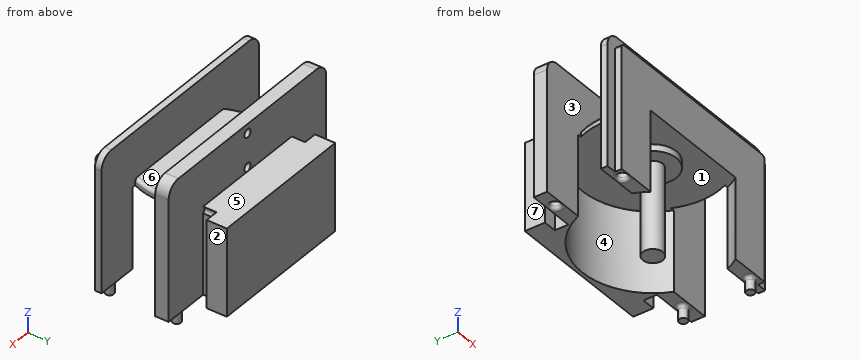
```python
from build123d import *

# Parameters (mm, degrees)
BOSS_EXTRUDE1_DEPTH     = 1
SKETCH2_R               = 1.475
BOSS_EXTRUDE2_DEPTH     = 14
SKETCH3_R               = 3.5
BOSS_EXTRUDE3_DEPTH     = 1
SKETCH4_W               = 2
SKETCH4_H               = 17
BOSS_EXTRUDE4_DEPTH     = 12
SKETCH5_W               = 18
SKETCH5_H               = 2
BOSS_EXTRUDE5_DEPTH     = 12
SKETCH6_W               = 13
SKETCH6_H               = 2
BOSS_EXTRUDE6_DEPTH     = 5
BOSS_EXTRUDE7_DEPTH     = 12
CUT_EXTRUDE1_DEPTH      = 24.366642891
SKETCH9_W               = 2.937742252
SKETCH9_H               = 8
CUT_EXTRUDE2_DEPTH      = 12
CUT_EXTRUDE11_START     = -12
SKETCH21_R              = 10.5
SKETCH21_R_2            = 3.5
CUT_EXTRUDE11_DEPTH     = 12
SKETCH10_W              = 32
SKETCH10_H              = 2
BOSS_EXTRUDE8_DEPTH     = 7
FILLET1_R               = 0.5
SKETCH11_R              = 0.625
BOSS_EXTRUDE9_DEPTH     = 2
SKETCH14_W              = 2
SKETCH14_H              = 2
CUT_EXTRUDE5_DEPTH      = 28.874719859
SKETCH12_R              = 0.675
CUT_EXTRUDE3_DEPTH      = 2.5
CUT_EXTRUDE6_DEPTH      = 2
FILLET2_R               = 0.5
FILLET3_R               = 0.5
FILLET4_R               = 2
CUT_EXTRUDE7_DEPTH      = 28.221315288
CUT_EXTRUDE7_DEPTH_BACK = 1
SKETCH19_R              = 0.625
CUT_EXTRUDE9_DEPTH      = 2


with BuildPart() as part:
    # Sketch1 → Boss-Extrude1 (new body)
    with BuildSketch(Plane.XY):
        Polygon((-11, 6), (-11, 11), (11, 11), (11, 6), (11, -6), (-11, -6), align=None)
    extrude(amount=BOSS_EXTRUDE1_DEPTH)

    # Sketch2 → Boss-Extrude2 (add)
    with BuildSketch(Plane(origin=(0, 0, 0), x_dir=(-1, 0, 0), z_dir=(0, 0, -1))):
        with Locations(Location((0, 0, 0), (0, 0, 180))):
            Circle(SKETCH2_R)
    extrude(amount=BOSS_EXTRUDE2_DEPTH)

    # Sketch3 → Boss-Extrude3 (add)
    with BuildSketch(Plane(origin=(0, 0, 0), x_dir=(-1, 0, 0), z_dir=(0, 0, -1))):
        with Locations(Location((0, 0, 0), (0, 0, 180))):
            Circle(SKETCH3_R)
    extrude(amount=BOSS_EXTRUDE3_DEPTH)

    # Sketch4 → Boss-Extrude4 (add)
    with BuildSketch(Plane(origin=(0, 0, 0), x_dir=(-1, 0, 0), z_dir=(0, 0, -1))):
        with Locations((10, 2.5)):
            Rectangle(SKETCH4_W, SKETCH4_H)
        with Locations((-10, 2.5)):
            Rectangle(SKETCH4_W, SKETCH4_H)
    extrude(amount=BOSS_EXTRUDE4_DEPTH)

    # Sketch5 → Boss-Extrude5 (add)
    with BuildSketch(Plane(origin=(0, 0, 0), x_dir=(-1, 0, 0), z_dir=(0, 0, -1))):
        with Locations((0, 10)):
            Rectangle(SKETCH5_W, SKETCH5_H)
    extrude(amount=BOSS_EXTRUDE5_DEPTH)

    # Sketch6 → Boss-Extrude6 (add)
    with BuildSketch(Plane(origin=(11, 0, 0), x_dir=(0, 0, -1), z_dir=(1, 0, 0))):
        with Locations((5.5, -5)):
            Rectangle(SKETCH6_W, SKETCH6_H)
        with Locations((5.5, 5)):
            Rectangle(SKETCH6_W, SKETCH6_H)
    boss_extrude6 = extrude(amount=BOSS_EXTRUDE6_DEPTH)

    # Mirror1: Boss-Extrude6 across plane
    add(boss_extrude6.mirror(Plane(origin=(0, 0, 0), x_dir=(0, 0, 1), z_dir=(1, 0, 0))))

    # Sketch7 → Boss-Extrude7 (add)
    with BuildSketch(Plane(origin=(0, 0, -12), x_dir=(-1, 0, 0), z_dir=(0, 0, -1))):
        with BuildLine():
            ThreePointArc((-6.708203932, -6), (-8.407551231, -3.211398808), (-9, 0))
            Line((-9, 0), (-9, -6))
            Line((-9, -6), (-6.708203932, -6))
        make_face()
        with BuildLine():
            Line((-9, 9), (-9, 0))
            ThreePointArc((-9, 0), (-6.363961031, 6.363961031), (0, 9))
            Line((0, 9), (-9, 9))
        make_face()
    boss_extrude7 = extrude(amount=-BOSS_EXTRUDE7_DEPTH)

    # Sketch8 → Cut-Extrude1 (cut, through all)
    with BuildSketch(Plane(origin=(0, 0, -12), x_dir=(-1, 0, 0), z_dir=(0, 0, -1))):
        with BuildLine():
            Line((-11, 4), (-9.16515139, 4))
            ThreePointArc((-9.16515139, 4), (-10, 0), (-9.16515139, -4))
            Line((-9.16515139, -4), (-11, -4))
            Line((-11, -4), (-11, 4))
        make_face()
    cut_extrude1 = extrude(amount=-CUT_EXTRUDE1_DEPTH, mode=Mode.SUBTRACT)

    # Sketch9 → Cut-Extrude2 (cut)
    with BuildSketch(Plane(origin=(0, 0, -12), x_dir=(-1, 0, 0), z_dir=(0, 0, -1))):
        with Locations((-9.531128874, 0)):
            Rectangle(SKETCH9_W, SKETCH9_H)
    cut_extrude2 = extrude(amount=-CUT_EXTRUDE2_DEPTH, mode=Mode.SUBTRACT)

    # Mirror2: Boss-Extrude7, Cut-Extrude1, Cut-Extrude2 across plane
    add(boss_extrude7.mirror(Plane(origin=(0, 0, 0), x_dir=(0, 0, 1), z_dir=(1, 0, 0))))
    add(cut_extrude1.mirror(Plane(origin=(0, 0, 0), x_dir=(0, 0, 1), z_dir=(1, 0, 0))), mode=Mode.SUBTRACT)
    add(cut_extrude2.mirror(Plane(origin=(0, 0, 0), x_dir=(0, 0, 1), z_dir=(1, 0, 0))), mode=Mode.SUBTRACT)

    # Sketch21 → Cut-Extrude11 (cut)
    with BuildSketch(Plane(origin=(0, 0, -12), x_dir=(-1, 0, 0), z_dir=(0, 0, -1)).offset(CUT_EXTRUDE11_START)):
        Circle(SKETCH21_R)
        with Locations(Location((0, 0, 0), (0, 0, 180))):
            Circle(SKETCH21_R_2, mode=Mode.SUBTRACT)
    extrude(amount=CUT_EXTRUDE11_DEPTH, mode=Mode.SUBTRACT)

    # Sketch10 → Boss-Extrude8 (add)
    with BuildSketch(Plane.XY.offset(1)):
        with Locations((0, -5)):
            Rectangle(SKETCH10_W, SKETCH10_H)
        with Locations((0, 5)):
            Rectangle(SKETCH10_W, SKETCH10_H)
    extrude(amount=BOSS_EXTRUDE8_DEPTH)

    # Fillet1
    fillet1_edges = [part.edges().sort_by_distance(p)[0] for p in [
        (10, 0, 1),
        (-10, 0, 1),
    ]]
    fillet(fillet1_edges, radius=FILLET1_R)

    # Sketch11 → Boss-Extrude9 (add)
    with BuildSketch(Plane(origin=(0, 0, -12), x_dir=(-1, 0, 0), z_dir=(0, 0, -1))):
        with Locations(Location((-13, -5, 0), (0, 0, 180))):
            Circle(SKETCH11_R)
    boss_extrude9 = extrude(amount=BOSS_EXTRUDE9_DEPTH)

    # Sketch14 → Cut-Extrude5 (cut, through all)
    with BuildSketch(Plane(origin=(0, 0, -12), x_dir=(-1, 0, 0), z_dir=(0, 0, -1))):
        with Locations((10, 7)):
            Rectangle(SKETCH14_W, SKETCH14_H)
        with Locations((-10, 7)):
            Rectangle(SKETCH14_W, SKETCH14_H)
    extrude(amount=-CUT_EXTRUDE5_DEPTH, mode=Mode.SUBTRACT)

    # Sketch12 → Cut-Extrude3 (cut)
    with BuildSketch(Plane(origin=(0, 0, -12), x_dir=(-1, 0, 0), z_dir=(0, 0, -1))):
        with Locations((13, -5)):
            Circle(SKETCH12_R)
    cut_extrude3 = extrude(amount=-CUT_EXTRUDE3_DEPTH, mode=Mode.SUBTRACT)

    # Sketch16 → Cut-Extrude6 (cut)
    with BuildSketch(Plane(origin=(0, 6, 0), x_dir=(1, 0, 0), z_dir=(0, 1, 0))):
        with BuildLine():
            Line((-9, 0), (-9, -1))
            ThreePointArc((-9, -1), (-8.75, -0.5), (-9, 0))
        make_face()
    cut_extrude6 = extrude(amount=CUT_EXTRUDE6_DEPTH, mode=Mode.SUBTRACT)

    # Mirror3: Boss-Extrude9, Cut-Extrude3 across plane
    add(boss_extrude9.mirror(Plane.ZX))
    add(cut_extrude3.mirror(Plane.ZX), mode=Mode.SUBTRACT)

    # Mirror4: Cut-Extrude6 across plane
    add(cut_extrude6.mirror(Plane(origin=(0, 0, 0), x_dir=(0, 0, 1), z_dir=(1, 0, 0))), mode=Mode.SUBTRACT)

    # Fillet2
    fillet2_edges = [part.edges().sort_by_distance(p)[0] for p in [
        (12.375, -5, -12),
        (12.375, 5, -12),
    ]]
    fillet(fillet2_edges, radius=FILLET2_R)

    # Fillet3
    # the kernel refuses this fillet: 0.5 mm, written as the material it takes off along each edge
    with BuildSketch(Plane(origin=(-13, -5, -12), x_dir=(-1, 0, 0), z_dir=(0, -1, 0))) as fillet3_piece_1:
        with BuildLine():
            CenterArc((0.675 + FILLET3_R, -FILLET3_R), FILLET3_R, 90, 90)
            Line((0.675, -FILLET3_R), (0.675, 0))
            Line((0.675, 0), (0.675 + FILLET3_R, 0))
        make_face()
    revolve(axis=Axis((-13, -5, -12), (0, 0, -1)), mode=Mode.SUBTRACT)
    with BuildSketch(Plane(origin=(-13, 5, -12), x_dir=(-1, 0, 0), z_dir=(0, 1, 0))) as fillet3_piece_2:
        with BuildLine():
            CenterArc((0.675 + FILLET3_R, FILLET3_R), FILLET3_R, 180, 90)
            Line((0.675, FILLET3_R), (0.675, 0))
            Line((0.675, 0), (0.675 + FILLET3_R, 0))
        make_face()
    revolve(axis=Axis((-13, 5, -12), (0, 0, 1)), mode=Mode.SUBTRACT)

    # Fillet4
    fillet4_edges = [part.edges().sort_by_distance(p)[0] for p in [
        (16, -5, 8),
        (-16, -5, 8),
        (-16, 5, 8),
        (16, 5, 8),
    ]]
    fillet(fillet4_edges, radius=FILLET4_R)

    # Sketch17 → Cut-Extrude7 (cut, two sides: drawn at the far end of the back side and taken through both)
    with BuildSketch(Plane.XZ.offset(6).offset(-CUT_EXTRUDE7_DEPTH_BACK)):
        with BuildLine():
            Line((-16, 6), (-16, -12))
            Line((-16, -12), (-14.5, -12))
            Line((-14.5, -12), (-14.5, 6))
            ThreePointArc((-14.5, 6), (-14.353553391, 6.353553391), (-14, 6.5))
            Line((-14, 6.5), (14, 6.5))
            ThreePointArc((14, 6.5), (14.353553391, 6.353553391), (14.5, 6))
            Line((14.5, 6), (14.5, -12))
            Line((14.5, -12), (16, -12))
            Line((16, -12), (16, 6))
            ThreePointArc((16, 6), (15.414213562, 7.414213562), (14, 8))
            Line((14, 8), (-14, 8))
            ThreePointArc((-14, 8), (-15.414213562, 7.414213562), (-16, 6))
        make_face()
    extrude(amount=CUT_EXTRUDE7_DEPTH + CUT_EXTRUDE7_DEPTH_BACK, mode=Mode.SUBTRACT)

    # Sketch19 → Cut-Extrude9 (cut)
    with BuildSketch(Plane(origin=(0, 6, 0), x_dir=(1, 0, 0), z_dir=(0, 1, 0))):
        with Locations(Location((0, -1.625, 0), (0, 0, 90))):
            Circle(SKETCH19_R)
        with Locations(Location((0, -6.625, 0), (0, 0, 270))):
            Circle(SKETCH19_R)
    extrude(amount=-CUT_EXTRUDE9_DEPTH, mode=Mode.SUBTRACT)


solid = part.part
```
CAD build for the part. Positions are in the model's coordinates, mm. Face numbers are marked on the shaded views. A direction names the side the tool comes from. Round coordinates to 2 decimals unless told otherwise and drop trailing zeros. Loops run counter-clockwise (first coordinate to the right, second up) from the corner with the lowest first, then second, coordinate; pieces in that order, holes last. Notation, with made-up numbers: M 79,69.25 L 122,69.25 A30 cw 122,95.25 Z; hole C 70.25,-4 d5. An arc over 180 degrees is marked long. Return JSON: item names as keys, results as strings. Group by question number.
(1) Wall check: probe 1 along Y at (x, z) = (-13, -10.75) (3 decimals); probe 2 along Y at (x, z) = (6.5, 5.75); probe 3 along X at (y, z) = (5, -11.1) (3 decimals). Give the ranges that are in metal, low to high. Write a range as [from, to].
(2) Saw through at B-B, the plane z = -2.25. List the corners of the cut face in (x, y) (3 decimals), and give its area (3 significant figures).
(3) Saw through at D-D, the plane y = 5. List the corners of the cut face in (x, z) (3 decimals), and give its area (3 significant figures).
(4) Saw through at C-C, the plane y = 0. List the corners of the cut face in (x, z) (3 decimals), and give its area (3 significant figures).
(5) Saw through at A-A, the plane x = 11.5. List the corners of the cut face in (y, z).
(6) Drop flat-ended pins along their axis: P1, Ø2, axis at x = -12, y = 0, coming from the -Z side (3 decimals); P2, Ø0.5, axis at x = -6.5, y = -5.5, coming from the +Z side; P3, Ø2, axis at x = 0, z = 1.625, coming from the +Y side; P4, Ø8, axis at x = 4, z = -4.5, coming from the -Y side. Give the stop position or say it passes through.
(7) Tool access for the marked faces 4, 5, 6 and 7: list every direction of +Z, -Z, +X, -X, +Y, -Y with a clear straight run to the whole face (end or side of a thin tool).
(8) Mould opens along X. For the marked faces 1, 2 and 3 say: +X half, -X half, draft (parallel to the pull), parting line (faces both ways), or undercut.
Answer list:
{
 "1": {"probe 1": "[-6, -5.675], [-4.325, -4], [4, 4.325], [5.675, 6]", "probe 2": "[-6, -4], [4, 6]", "probe 3": "[-16, -13.675], [-12.325, -9.233], [9.233, 16]"},
 "2": {"outline": "M -16,-5 L -14.5,-5 L -14.5,-6 L -8.617,-6 A10.5 cw -9.708,-4 L -16,-4 Z; M -16,4 L -9.708,4 A10.5 cw 9.708,4 L 16,4 L 16,6 L 9,6 L 9,8 L 11,8 L 11,11 L -11,11 L -11,8 L -9,8 L -9,6 L -16,6 Z; C 0,0 d2.95; M 8.617,-6 L 14.5,-6 L 14.5,-5 L 16,-5 L 16,-4 L 9.708,-4 A10.5 cw Z", "area": "106 mm2"},
 "3": {"outline": "M -16,-12 L -14.175,-12 A0.5 ccw -13.675,-11.5 L -13.675,-9.5 L -12.325,-9.5 L -12.325,-11.5 A0.5 ccw -11.825,-12 L -9.233,-12 L -9.233,0 L 9.233,0 L 9.233,-12 L 11.875,-12 A0.5 cw 12.375,-12.5 L 12.375,-14 L 13.625,-14 L 13.625,-12.5 A0.5 cw 14.125,-12 L 16,-12 L 16,6 A2 ccw 14,8 L -14,8 A2 ccw -16,6 Z; hole C 0,1.625 d1.25; hole C 0,6.625 d1.25", "area": "413 mm2"},
 "4": {"outline": "M -10,0 L -3.5,0 L -3.5,-1 L -1.475,-1 L -1.475,-14 L 1.475,-14 L 1.475,-1 L 3.5,-1 L 3.5,0 L 10,0 L 10,0.5 A0.5 ccw 9.5,1 L -9.5,1 A0.5 ccw -10,0.5 Z", "area": "65.2 mm2"},
 "5": {"outline": "M -6,-12 L -4,-12 L -4,8 L -5,8 L -5,6.5 L -6,6.5 Z; M 4,-12 L 6,-12 L 6,8 L 4,8 Z"},
 "6": {"P1": "through", "P2": "z = 6.5", "P3": "y = 11", "P4": "y = -2.83"},
 "7": {"face 4": "-Z", "face 5": "+Z, +X, -X, +Y", "face 6": "+Z, +X, -X", "face 7": "+Z, -Z, -X, +Y"},
 "8": {"face 1": "undercut", "face 2": "+X half", "face 3": "draft"}
}
